Build history of the part. All positions in model axes, mm. A direction names the side the tool comes from. Give positions to 0.01 mm unless a question says otherwise; leave off trailing zeros. Order: outer loops, then holes, each group sorted by start corner. A loop starts at its lowest first (then second) coordinate and runs counter-clockwise, first axis right, second up. Notation, with made-up numbers: (41.25, -32.5) -> (51.25, -32.5) arc R25 cw to (51.25, 2.5) -> close; hole circle Ø9 at (-20.75, -20). An arc over 180 degrees is marked (long way). Write item = value, one per line. Start each with the question number.
from build123d import *

# Parameters (mm, degrees)
F1_DEPTH = 5
F0_R     = 1.5
F2_DEPTH = 25


with BuildPart() as f1:
    # F0 (on Top) → F1 (new body)
    with BuildSketch(Plane.XY):
        with BuildLine():
            Line((-4.5315389352, -6.4717082978), (-86.0364654527, -122.8728066433))
            Line((-86.0364654527, -122.8728066433), (-81.9407052312, -125.7406888251))
            Line((-81.9407052312, -125.7406888251), (-0.4357787137, -9.3395904795))
            ThreePointArc((-0.4357787137, -9.3395904795), (-2.8678821818, -8.4543772105), (-4.5315389352, -6.4717082978))
        make_face()
        Polygon((-86.0364654527, -122.8728066433), (-94.2279858955, -117.1370422798), (-108.5673968043, -137.6158433871), (-88.0885956971, -151.9552542958), (-73.7491847883, -131.4764531886), (-81.9407052312, -125.7406888251), align=None)
    extrude(amount=F1_DEPTH)



with BuildPart() as f1b:
    # F0 (on Top) → F1, piece 2 (new body)
    with BuildSketch(Plane.XY):
        with BuildLine():
            ThreePointArc((4.5315389352, -6.4717082978), (2.8678821818, -8.4543772105), (0.4357787137, -9.3395904795))
            Line((0.4357787137, -9.3395904795), (81.9407052312, -125.7406888251))
            Line((81.9407052312, -125.7406888251), (86.0364654527, -122.8728066433))
            Line((86.0364654527, -122.8728066433), (4.5315389352, -6.4717082978))
        make_face()
        Polygon((86.0364654527, -122.8728066433), (81.9407052312, -125.7406888251), (73.7491847883, -131.4764531886), (88.0885956971, -151.9552542958), (108.5673968043, -137.6158433871), (94.2279858955, -117.1370422798), align=None)
    extrude(amount=F1_DEPTH)


with BuildPart() as f1_1:
    add(f1.part)

    add(f1b.part)  # F2 merges F1b
    # F0 (on Top) → F2 (join)
    with BuildSketch(Plane.XY):
        with BuildLine():
            ThreePointArc((5, -4.3586169891), (-1.0821980697, 0.5228630465), (-4.5315389352, -6.4717082978))
            ThreePointArc((-4.5315389352, -6.4717082978), (-2.8678821818, -8.4543772105), (-0.4357787137, -9.3395904795))
            ThreePointArc((-0.4357787137, -9.3395904795), (0, -9.3586169891), (0.4357787137, -9.3395904795))
            ThreePointArc((0.4357787137, -9.3395904795), (2.8678821818, -8.4543772105), (4.5315389352, -6.4717082978))
            ThreePointArc((4.5315389352, -6.4717082978), (4.8814800356, -5.4408150587), (5, -4.3586169891))
        make_face()
        with Locations((0, -4.3586169891)):
            Circle(F0_R, mode=Mode.SUBTRACT)
    extrude(amount=F2_DEPTH)


solid = f1_1.part
(1) Cut at C-C, the plane x = -9. Give the cut face in (y, z), plus the area to 3 significant figures.
(2) Wall check: line 1 (Y direction, x = 0, z = 11); line 2 (Z direction, x = 70, y = -102.5); line 3 (X direction, y = -138.5, z = 4.5). Give the ranges that are in metal, low to high. Write a range as [from, to].
(3) Cut at B-B, the plane z = 22.25. Give the cut face in (x, y).
(4) Mould opens along Y. For faces 1 (the face through (-67, -100, 5)), 2 (the face through (90.19, -119.965, 2.465)), 3 (the face through (-77.788, -128.649, 2.465)) say: released by +Y, released by -Y, zero draft, split by the parting line, or undercut.
(5) 3-axis set-ups, long thin cutter, end or side, ignore diameter. For faces 4 (the face through (-81.02, -141.86, 2.46)), 5 (the face through (77.9, -128.57, 2.46)), 6 (the face through (-90.07, -120.05, 2.46)): which of +Z, -Z, +X, -X, +Y, -Y reach the whole face in a straight line?
(6) Cut at A-A, the plane y = -60.5. Give the cut face in (x, z).
Results:
q1.outline = (-21.57, 0) -> (-12.85, 0) -> (-12.85, 5) -> (-21.57, 5) -> close
q1.area = 43.6 mm2
q2.line_1 = [-9.36, -5.86], [-2.86, 0.64]
q2.line_2 = [0, 5]
q2.line_3 = [-107.3, -78.67], [78.67, 107.3]
q3.outline = circle Ø10 at (0, -4.36); hole circle Ø3 at (0, -4.36)
q4.face_1 = zero draft
q4.face_2 = released by +Y
q4.face_3 = undercut
q5.face_4 = +Z, -Z, -Y
q5.face_5 = +Z, -Z
q5.face_6 = +Z, -Z, +Y
q6.outline = (-42.36, 0) -> (-36.26, 0) -> (-36.26, 5) -> (-42.36, 5) -> close; (36.26, 0) -> (42.36, 0) -> (42.36, 5) -> (36.26, 5) -> close
